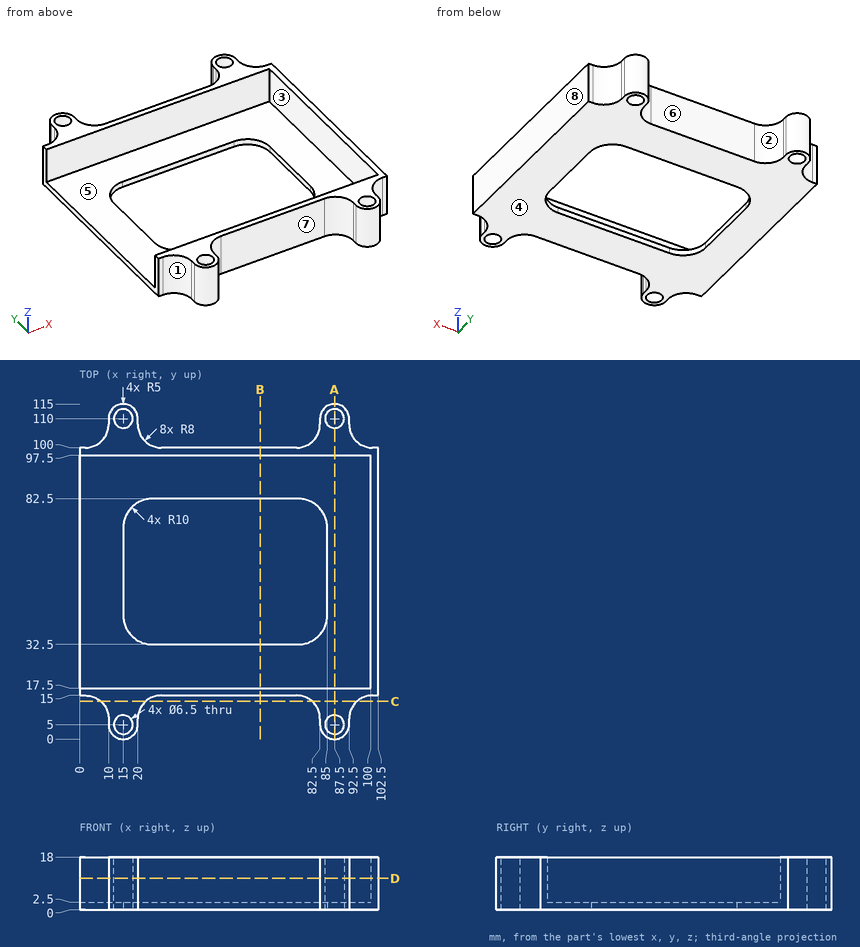
Design review of the part shown in the three views and the two pictorial views. Dimensions are in mm from the part's minimum x, y and z. A direction names the side the tool comes from. Round coordinates to 2 decimals unless told otherwise and drop trailing zeros. Write each loop counter-clockwise with the first axis right and the second up, starting at its lowest first coordinate (ties: lowest second). Pieces come first, ordered by that corner, then holes.
Item 1: For probe 1 along Y at (x, z) = (87.5, 12.75); probe 2 along Y at (x, z) = (12, 7.25); probe 3 along X at (y, z) = (8, 11.25), list the stretches that pass through material, from the lowest coordinate up.
Item 2: We need section B-B on x = 62. Write out the cut boundary in (y, z).
Item 3: The part is to be moulded in two halves that separate along Y. For the marked faces 1, 2 and 3, say which applies: +Y half, -Y half, draft (parallel to the pull), parting line (faces both ways), or undercut.
Item 4: Clearance check with flat-ended pins moving along their axes: pin 1 Ø1 at (x, z) = (10.5, 5) entering from +Y; pin 2 Ø1.6 at (y, z) = (108.5, 10) entering from +X; pin 3 Ø3 at (x, z) = (63, 5.5) entering from +Y; pin 4 Ø10 at (x, y) = (73, 76.5) entering from -Z. State where each tip first meets the part, or that it passes through.
Item 5: We need section A-A on x = 87.5. Write out the cut boundary in (y, z), and give its area (3 significant figures).
Item 6: We need section D-D on z = 10.75. State how many separate pieces and enclosed holes the cut face has, and give its area (3 significant figures).
Item 7: We need section C-C on y = 13. Write out the cut boundary in (x, z), and give its area (3 significant figures).
Item 8: For the marked faces 4, 5, 6, 7 and 8, list the 3-axis set-ups (+Z, -Z, +X, -X, +Y, -Y) from which the entire face can be reached by the end or side of a thin tool; tool diameter is ignored.
Returned:
1. probe 1: y = 0 to 1.75, 8.25 to 17.5, 97.5 to 106.75, 113.25 to 115
1. probe 2: y = 1 to 3.75, 6.25 to 17.5, 97.5 to 108.75, 111.25 to 114
1. probe 3: x = 9.94 to 13.75, 16.25 to 20.06, 82.44 to 86.25, 88.75 to 92.56
2. outline: (15, 0) - (32.5, 0) - (32.5, 2.5) - (17.5, 2.5) - (17.5, 18) - (15, 18) - close; (82.5, 0) - (100, 0) - (100, 18) - (97.5, 18) - (97.5, 2.5) - (82.5, 2.5) - close
3. face 1: -Y half
3. face 2: +Y half
3. face 3: undercut
4. pin 1: stops at y = 113
4. pin 2: stops at x = 92.51
4. pin 3: stops at y = 100
4. pin 4: passes through
5. outline: (0, 0) - (1.75, 0) - (1.75, 18) - (0, 18) - close; (8.25, 0) - (106.75, 0) - (106.75, 18) - (97.5, 18) - (97.5, 2.5) - (17.5, 2.5) - (17.5, 18) - (8.25, 18) - close; (113.25, 0) - (115, 0) - (115, 18) - (113.25, 18) - close
5. area: 596 mm2
6. separate pieces: 1
6. enclosed holes: 4
6. area: 1,250 mm2
7. outline: (7.29, 0) - (22.71, 0) - (22.71, 18) - (7.29, 18) - close; (79.79, 0) - (95.21, 0) - (95.21, 18) - (79.79, 18) - close
7. area: 555 mm2
8. face 4: -Z, +X, -X, +Y, -Y
8. face 5: +Z, -X
8. face 6: +Z, -Z, +Y
8. face 7: +Z, -Z, -Y
8. face 8: +Z, -Z, +X, +Y, -Y
